```python
from build123d import *

# Parameters (mm, degrees)
F1_DEPTH  = 32
F3_DEPTH  = 25
F5_DEPTH  = 25
F7_DEPTH  = 19
F9_DEPTH  = 19
F10_R     = 6.5
F11_DEPTH = 100
F12_R     = 5.5
F13_DEPTH = 25
F14_R     = 5.5
F15_DEPTH = 25


with BuildPart() as f1:
    # F0 (on Front) → F1 (new body)
    with BuildSketch(Plane.XZ):
        Polygon((0, 13), (0, 0), (39, 0), (39, 17), (74, 17), (74, 0), (113, 0), (113, 13), (88, 13), (88, 30), (39, 30), (25, 30), (25, 13), align=None)
    extrude(amount=-F1_DEPTH)

    # F2 (on face) → F3 (cut)
    with BuildSketch(Plane.XY.offset(13)):
        Polygon((113, 10), (103, 0), (113, 0), align=None)
    extrude(amount=-F3_DEPTH, mode=Mode.SUBTRACT)

    # F4 (on face) → F5 (cut)
    with BuildSketch(Plane.XY.offset(13)):
        Polygon((0, 0), (10, 0), (0, 10), align=None)
    extrude(amount=-F5_DEPTH, mode=Mode.SUBTRACT)

    # F6 (on face) → F7 (join)
    with BuildSketch(Plane.YZ.offset(88)):
        with BuildLine():
            Line((0, 60.128765), (0, 30))
            Line((0, 30), (32, 30))
            Line((32, 30), (32, 60.128765))
            ThreePointArc((32, 60.128765), (16, 64), (0, 60.128765))
        make_face()
    extrude(amount=-F7_DEPTH)

    # F8 (on face) → F9 (join)
    with BuildSketch(Plane(origin=(25, 0, 0), x_dir=(0, -1, 0), z_dir=(-1, 0, 0))):
        with BuildLine():
            Line((-32, 60.128765), (-32, 30))
            Line((-32, 30), (0, 30))
            Line((0, 30), (0, 60.128765))
            ThreePointArc((0, 60.128765), (-16, 64), (-32, 60.128765))
        make_face()
    extrude(amount=-F9_DEPTH)

    # F10 (on face) → F11 (cut)
    with BuildSketch(Plane.YZ.offset(88)):
        with Locations((16, 46)):
            Circle(F10_R)
    extrude(amount=-F11_DEPTH, mode=Mode.SUBTRACT)

    # F12 (on face) → F13 (cut)
    with BuildSketch(Plane.XY.offset(13)):
        with Locations((100, 19)):
            Circle(F12_R)
    extrude(amount=-F13_DEPTH, mode=Mode.SUBTRACT)

    # F14 (on face) → F15 (cut)
    with BuildSketch(Plane.XY.offset(13)):
        with Locations((13, 19)):
            Circle(F14_R)
    extrude(amount=-F15_DEPTH, mode=Mode.SUBTRACT)


solid = f1.part
```
For this review, take the finished solid that the model builds, in its own axes (mm). A direction names the side the tool comes from. Coordinates: 2 decimals unless noted, no trailing zeros. Loops run counter-clockwise (first coordinate to the right, second up) from the corner with the lowest first, then second, coordinate; pieces in that order, holes last.
1. For line 1 (X direction, y = 16.5, z = 39); line 2 (Y direction, x = 100, z = 9); line 3 (X direction, y = 18, z = 10), list the stretches that pass through material, from the lowest coordinate up.
2. Add section B-B, the plane z = 36.5. Give the boundary of the cut face in (x, y), then the cut area to 3 significant figures.
3. Add section C-C, the plane x = 13. Give the boundary of the cut face in (y, z), then the cut area to 3 significant figures.
4. For faces 1 (the flat face through (74, 16, 9)), 2 (the cylindrical face through (34.633, 10.842, 42.045)), 3 (the cylindrical face through (18.246, 20.652, 6.591)), 4 (the flat face through (101, 12, 13)), 5 (the flat face through (25, 16, 39)), list the 3-axis set-ups (+Z, -Z, +X, -X, +Y, -Y) from which the entire face can be reached by the end or side of a thin tool; tool diameter is ignored.
5. Insertion check: P1, Ø12.5, axis at x = 11.5, y = 22, coming from the +Z side; P2, Ø2, axis at x = 48.5, y = 7.5, coming from the +Z side; P3, Ø9.5, axis at y = 24, z = 48.5, coming from the -X side. Each pin has a flat end and moves straight along its axis. Give the tip position at first contact, or say it passes through.
6. Mouldability with a two-part tool opening along Y and no side actions: class faces 6 (the flat face through (56, 16, 17)), 7 (the flat face through (108, 5, 7)), 8 (the cylindrical face through (78.633, 10.842, 42.045)), 9 (the cylindrical face through (94.505, 19.242, 6.591)) as +Y half, -Y half, draft (parallel to the pull), parting line (faces both ways), or undercut.
7. Add section D-D, the plane y = 19. Count the separate pieces of the cut face and the enclosed holes in it, then the cut area to 3 significant figures.
8. Add section A-A, the plane z = 46. Give the boundary of the cut face in (x, y).
Result:
1. line 1: x = 25 to 44, 69 to 88
1. line 2: y = 0 to 13.5, 24.5 to 32
1. line 3: x = 0 to 7.59, 18.41 to 39, 74 to 94.59, 105.41 to 113
2. outline: (25, 0) - (44, 0) - (44, 32) - (25, 32) - close; (69, 0) - (88, 0) - (88, 32) - (69, 32) - close
2. area: 1,220 mm2
3. outline: (0, 0) - (13.5, 0) - (13.5, 13) - (0, 13) - close; (24.5, 0) - (32, 0) - (32, 13) - (24.5, 13) - close
3. area: 273 mm2
4. face 1: -Z, +Y, -Y
4. face 2: +X, -X
4. face 3: +Z, -Z
4. face 4: +Z, +X, +Y, -Y
4. face 5: +Z, -X, +Y, -Y
5. P1: stops at z = 13
5. P2: stops at z = 30
5. P3: stops at x = 25
6. face 6: draft
6. face 7: -Y half
6. face 8: undercut
6. face 9: undercut
7. separate pieces: 5
7. enclosed holes: 0
7. area: 2,510 mm2
8. outline: (25, 0) - (44, 0) - (44, 9.5) - (25, 9.5) - close; (25, 22.5) - (44, 22.5) - (44, 32) - (25, 32) - close; (69, 0) - (88, 0) - (88, 9.5) - (69, 9.5) - close; (69, 22.5) - (88, 22.5) - (88, 32) - (69, 32) - close
